```python
from build123d import *

# Parameters (mm, degrees)
SKETCH1_W            = 1208
SKETCH1_H            = 387
BOSS_EXTRUDE1_DEPTH  = 608
SKETCH2_W            = 1200
SKETCH2_H            = 379
CUT_EXTRUDE1_DEPTH   = 604
FILLET1_R            = 8
CUT_EXTRUDE2_DEPTH   = 2
MIRROR2_COPY_1_DEPTH = 2
SKETCH5_R            = 10
SKETCH5_W            = 40
SKETCH5_H            = 10
CUT_EXTRUDE4_DEPTH   = 4


with BuildPart() as part:
    # Sketch1 → Boss-Extrude1 (new body)
    with BuildSketch(Plane.XY):
        Rectangle(SKETCH1_W, SKETCH1_H)
    extrude(amount=BOSS_EXTRUDE1_DEPTH)

    # Sketch2 → Cut-Extrude1 (cut)
    with BuildSketch(Plane.XY.offset(608)):
        Rectangle(SKETCH2_W, SKETCH2_H)
    extrude(amount=-CUT_EXTRUDE1_DEPTH, mode=Mode.SUBTRACT)

    # Fillet1
    fillet1_edges = [part.edges().sort_by_distance(p)[0] for p in [
        (-604, 0, 0),
        (604, 0, 0),
    ]]
    fillet(fillet1_edges, radius=FILLET1_R)

    # Sketch4 → Cut-Extrude2 (cut)
    with BuildSketch(Plane(origin=(0, 193.5, 0), x_dir=(1, 0, 0), z_dir=(0, 1, 0))):
        Polygon((-600, -604), (-588, -604), (-588, -602), (-598, -602), (-598, -592), (-600, -592), align=None)
    cut_extrude2 = extrude(amount=-CUT_EXTRUDE2_DEPTH, mode=Mode.SUBTRACT)

    # Mirror1: Cut-Extrude2 across plane
    add(cut_extrude2.mirror(Plane(origin=(0, 0, 0), x_dir=(0, 0, 1), z_dir=(1, 0, 0))), mode=Mode.SUBTRACT)

    # Mirror2: Cut-Extrude2 across plane
    add(cut_extrude2.mirror(Plane.XY.offset(304)), mode=Mode.SUBTRACT)

    # Mirror2 copy 1 sketch → Mirror2 copy 1 (cut)
    with BuildSketch(Plane(origin=(0, 193.5, 608), x_dir=(-1, 0, 0), z_dir=(0, 1, 0))):
        Polygon((-600, -604), (-588, -604), (-588, -602), (-598, -602), (-598, -592), (-600, -592), align=None)
    extrude(amount=-MIRROR2_COPY_1_DEPTH, mode=Mode.SUBTRACT)

    # Sketch5 → Cut-Extrude4 (cut)
    with BuildSketch(Plane(origin=(0, 193.5, 0), x_dir=(1, 0, 0), z_dir=(0, 1, 0))):
        with Locations((-100, -29)):
            Circle(SKETCH5_R)
        with Locations((530, -27)):
            Circle(SKETCH5_R)
        with Locations((-520, -27)):
            Rectangle(SKETCH5_W, SKETCH5_H)
    extrude(amount=-CUT_EXTRUDE4_DEPTH, mode=Mode.SUBTRACT)


solid = part.part
```
Could you check a few things on this model? Use its own coordinates, in mm. A direction names the side the tool comes from. Coordinates: 2 decimals unless noted, no trailing zeros. Loops run counter-clockwise (first coordinate to the right, second up) from the corner with the lowest first, then second, coordinate; pieces in that order, holes last.
1) Please list where these lines run through material, in increasing order: line 1 along X through (y, z) = (190.45, 27); line 2 along Y through (x, z) = (247.5, 554.5); line 3 along X through (y, z) = (10, 453.5).
Reported:
line 1: x = -604 to -540, -500 to -109.8, -90.2 to 520, 540 to 604
line 2: y = -193.5 to -189.5, 189.5 to 193.5
line 3: x = -604 to -600, 600 to 604
2) Imagine slicing it at B-B (y = -118.5). List the corners of the cut face in (x, z) for me.
Reported:
outline: (-604, 8) arc R8 ccw to (-596, 0) - (596, 0) arc R8 ccw to (604, 8) - (604, 608) - (600, 608) - (600, 4) - (-600, 4) - (-600, 608) - (-604, 608) - close
3) Imagine slicing it at C-C (x = 337.5). List the corners of the cut face in (y, z) for me, and give its area (3 significant figures).
Reported:
outline: (-193.5, 0) - (193.5, 0) - (193.5, 608) - (189.5, 608) - (189.5, 4) - (-189.5, 4) - (-189.5, 608) - (-193.5, 608) - close
area: 6,380 mm2
4) Imagine slicing it at A-A (z = 292). List the corners of the cut face in (x, y) for me, and give its area (3 significant figures).
Reported:
outline: (-604, -193.5) - (604, -193.5) - (604, 193.5) - (-604, 193.5) - close; hole (-600, -189.5) - (600, -189.5) - (600, 189.5) - (-600, 189.5) - close
area: 12,700 mm2
5) Which directions (+Z, -Z, +X, -X, +Y, -Y) give clear straight access to the entire face, cutting with the end or side of a thin tool? Please do faces 4 (the face through (600, -3, 310)), 5 (the face through (-8, 193.5, 300)).
Reported:
face 4: +Z
face 5: +Z, -Z, +X, -X, +Y
6) Thinking about a two-plate mould opening in X: for faces 1 (the face through (-8, 3, 0)), 2 (the face through (604, -3, 304)), 3 (the face through (-8, 189.5, 310)), which applies, released by +X, released by -X, zero draft, split by the parting line, or undercut?
Reported:
face 1: zero draft
face 2: released by +X
face 3: undercut
7) Will these pins go through, and if not, where does the flat tip stop? pin 1 Ø2 at (y, z) = (192.5, 5) entering from +X; pin 2 Ø2 at (y, z) = (192.5, 5.5) entering from -X; pin 3 Ø4 at (x, y) = (-442, -147.5) entering from +Z.
Reported:
pin 1: stops at x = 603.75
pin 2: stops at x = -603.86
pin 3: stops at z = 4
